Here's how the part is built. I have some questions about the finished solid (model axes, mm). Face numbers are marked on the shaded views. A direction names the side the tool comes from. Coordinates: 2 decimals unless noted, no trailing zeros. Write each loop counter-clockwise with the first axis right and the second up, starting at its lowest first coordinate (ties: lowest second). Pieces come first, ordered by that corner, then holes.
Solid Edge part; units mm, degrees
sketch "Sketch1" plane through (0, 0, 0) normal (0, 0, 1) x (1, 0, 0)
  line L0 (11.5, -10) -> (11.5, 10)
  line L1 (11.5, 10) -> (-11.5, 10)
  line L2 (-11.5, 10) -> (-11.5, -10)
  line L3 (-11.5, -10) -> (11.5, -10)
extrude "Protrusion1" add sketch "Sketch1" along normal mid plane 1.6
sketch "Sketch2" plane through (0, 0, 0.8) normal (0, 0, 1) x (1, 0, 0)
  line L0 (7.5, -7.5) -> (7.5, 7.5)
  line L1 (7.5, 7.5) -> (-7.5, 7.5)
  line L2 (-7.5, 7.5) -> (-7.5, -7.5)
  line L3 (-7.5, -7.5) -> (7.5, -7.5)
extrude "ExtrudedCutout_1" add sketch "Sketch2" along normal blind 5
sketch "Sketch3" plane through (0, 0, 5.8) normal (0, 0, 1) x (1, 0, 0)
  line L0 (1, -3.25) -> (-1, -3.25)
  line L1 (-1, -3.25) -> (-1, -2.25)
  line L2 (-1, -2.25) -> (1, -2.25)
  line L3 (1, -2.25) -> (1, -3.25)
  line L4 (-5.125, -2.25) -> (5.125, -2.25)
  line L5 (5.125, -2.25) -> (5.125, 2.25)
  line L6 (5.125, 2.25) -> (-5.125, 2.25)
  line L7 (-5.125, 2.25) -> (-5.125, -2.25)
extrude "ExtrudedProtrusion_3" add sketch "Sketch3" along normal blind 3
sketch "Sketch4" plane through (0, 0, 5.8) normal (0, 0, 1) x (1, 0, 0)
  line L0 (1, -2.25) -> (1, -3.25)
  line L1 (1, -3.25) -> (-1, -3.25)
  line L2 (-1, -3.25) -> (-1, -2.25)
  line L3 (-5.125, -2.25) -> (-1, -2.25)
  line L4 (-5.125, 2.25) -> (-5.125, -2.25)
  line L5 (5.125, 2.25) -> (-5.125, 2.25)
  line L6 (5.125, -2.25) -> (5.125, 2.25)
  line L7 (1, -2.25) -> (5.125, -2.25)
  line L8 (1.875, -4.125) -> (1.875, -3.125)
  line L9 (1.875, -3.125) -> (6, -3.125)
  line L10 (6, -3.125) -> (6, 3.125)
  line L11 (6, 3.125) -> (-6, 3.125)
  line L12 (-6, 3.125) -> (-6, -3.125)
  line L13 (-6, -3.125) -> (-1.875, -3.125)
  line L14 (-1.875, -3.125) -> (-1.875, -4.125)
  line L15 (-1.875, -4.125) -> (1.875, -4.125)
extrude "ExtrudedProtrusion_4" add sketch "Sketch4" along normal blind 0.5
sketch "Sketch5" plane through (0, -0.5, 8.8) normal (0, 0, 1) x (1, 0, 0)
  line L0 (-3.4, 1.9) -> (-3.4, -0.9)
  line L1 (-3.4, -0.9) -> (-2.4, -0.9)
  line L2 (-2.4, -0.9) -> (-2.4, 1.9)
  line L3 (-2.4, 1.9) -> (-3.4, 1.9)
  line L4 (3.4, -0.9) -> (3.4, 1.9)
  line L5 (3.4, 1.9) -> (2.4, 1.9)
  line L6 (2.4, 1.9) -> (2.4, -0.9)
  line L7 (2.4, -0.9) -> (3.4, -0.9)
extrude "Cutout1" cut sketch "Sketch5" against normal up to vertex (3 mm away)
sketch "Sketch6" plane through (0, 0, -0.8) normal (0, 0, -1) x (0, -1, 0)
  line L0 (10, 11.5) -> (10, -11.5)
  line L1 (10, -11.5) -> (-10, -11.5)
  line L2 (-10, -11.5) -> (-10, 11.5)
  line L3 (-10, 11.5) -> (10, 11.5)
extrude "Cutout2" cut sketch "Sketch6" against normal up to vertex (1.6 mm away)
sketch "Sketch7" plane through (0, 0, 0.8) normal (0, 0, -1) x (-1, 0, 0)
  circle A0 centre (-5.5, 0) radius 0.8
  circle A1 centre (0, 0) radius 1.6
  circle A2 centre (5.5, 0) radius 0.8
extrude "ExtrudedProtrusion_5" add sketch "Sketch7" along normal blind 2.5
sketch "Sketch8" plane through (0, 0, 0.8) normal (0, 0, -1) x (1, 0, 0)
  line L0 (-0.45, 6) -> (0.45, 6)
  line L1 (0.45, 6) -> (0.45, 6.25)
  line L2 (0.45, 6.25) -> (-0.45, 6.25)
  line L3 (-0.45, 6.25) -> (-0.45, 6)
  line L4 (-4.85, 3.75) -> (-5.75, 3.75)
  line L5 (-5.75, 3.75) -> (-5.75, 3.5)
  line L6 (-5.75, 3.5) -> (-4.85, 3.5)
  line L7 (-4.85, 3.5) -> (-4.85, 3.75)
extrude "ExtrudedProtrusion_6" add sketch "Sketch8" along normal blind 3.5
properties material "Polycarbonate"
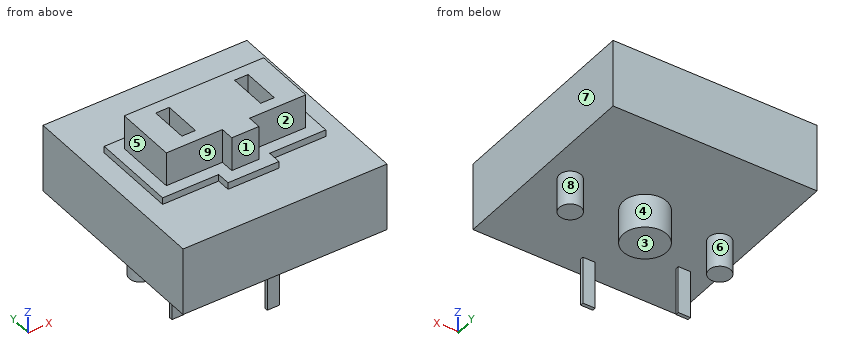
1. For pin 1 Ø2 at (y, z) = (0, 7.5) entering from +X (3 decimals); pin 2 Ø2 at (x, z) = (2, 7) entering from -Y (3 decimals); pin 3 Ø2 at (x, z) = (1, 7) entering from +Y (3 decimals); pin 4 Ø5 at (y, z) = (4, 7) entering from +X, each with a flat end and sliding along its axis, tell me the tip position at first contact or that it passes through.
2. If I drill on line 1 (X direction, y = 0.25, z = 8) (3 decimals); line 2 (Z direction, x = 0.5, y = 1.25); line 3 (Y direction, x = -5.5, z = 6) (3 decimals), over which ranges is the centre line in solid material (lowest first)?
3. Thinking about a two-plate mould opening in Y: for the marked faces 6, 7, 8 and 9, which applies, pulls with the +Y half, pulls with the -Y half, needs draft (parallel to the pull), parting line crosses it, or undercut?
4. On a 3-axis mill with a long thin cutter (end or side, diameter ignored), from which of +Z, -Z, +X, -X, +Y, -Y can I reach the whole of each face in a straight line? I mean the marked faces 1, 2, 3, 4 and 5. Say none if no direction works.
5. I want a section at D-D (z = 8). List the corners of the cut face in (x, y) for me (3 decimals).
6. I want a section at A-A (z = 0.25). List the corners of the cut face in (x, y) for me.
7. I want a section at B-B (x = 0). List the corners of the cut face in (y, z) for me (3 decimals), then the cut area to 3 significant figures.
Response values:
1. pin 1: stops at x = 5.125
1. pin 2: stops at y = -4.125
1. pin 3: stops at y = 3.125
1. pin 4: stops at x = 7.5
2. line 1: x = -5.125 to -3.4, -2.4 to 2.4, 3.4 to 5.125
2. line 2: z = -1.7 to 8.8
2. line 3: y = -3.125 to 3.125
3. face 6: undercut
3. face 7: needs draft
3. face 8: parting line crosses it
3. face 9: pulls with the -Y half
4. face 1: +Z, +X, -X, -Y
4. face 2: +Z, +X, -Y
4. face 3: -Z, +X, -X, +Y
4. face 4: -Z
4. face 5: +Z, -X, +Y, -Y
5. outline: (-5.125, -2.25) - (-1, -2.25) - (-1, -3.25) - (1, -3.25) - (1, -2.25) - (5.125, -2.25) - (5.125, 2.25) - (-5.125, 2.25) - close; hole (-3.4, -1.4) - (-2.4, -1.4) - (-2.4, 1.4) - (-3.4, 1.4) - close; hole (2.4, -1.4) - (3.4, -1.4) - (3.4, 1.4) - (2.4, 1.4) - close
6. outline: circle Ø1.6 at (-5.5, 0); (-5.75, -3.75) - (-4.85, -3.75) - (-4.85, -3.5) - (-5.75, -3.5) - close; circle Ø3.2 at (0, 0); (-0.45, -6.25) - (0.45, -6.25) - (0.45, -6) - (-0.45, -6) - close; circle Ø1.6 at (5.5, 0)
7. outline: (-7.5, 0.8) - (-6.25, 0.8) - (-6.25, -2.7) - (-6, -2.7) - (-6, 0.8) - (-1.6, 0.8) - (-1.6, -1.7) - (1.6, -1.7) - (1.6, 0.8) - (7.5, 0.8) - (7.5, 5.8) - (3.125, 5.8) - (3.125, 6.3) - (2.25, 6.3) - (2.25, 8.8) - (-3.25, 8.8) - (-3.25, 6.3) - (-4.125, 6.3) - (-4.125, 5.8) - (-7.5, 5.8) - close
7. area: 101 mm2
